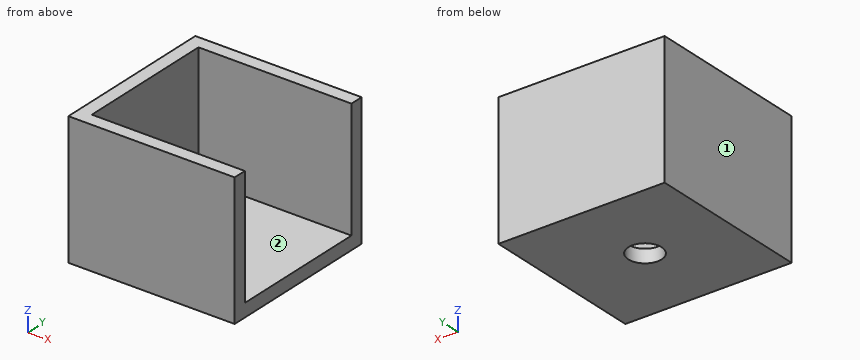
```python
from build123d import *

# Parameters (mm, degrees)
IZIM1_W                     = 25
IZIM1_H                     = 25
Y_KSEKLIK_EKSTR_ZYON1_DEPTH = 20
BO_ALTMA1_T                 = -2
IZIM2_R                     = 2.5
KES_EKSTR_ZYON1_DEPTH       = 5


with BuildPart() as part:
    # Çizim1 → Yükseklik-Ekstrüzyon1 (new body)
    with BuildSketch(Plane.XY):
        Rectangle(IZIM1_W, IZIM1_H)
    extrude(amount=Y_KSEKLIK_EKSTR_ZYON1_DEPTH)

    # İç Boşaltma1
    bo_altma1_openings = [part.faces().sort_by_distance(p)[0] for p in [
        (0, 0, 20),
        (12.5, 0, 10),
    ]]
    offset(amount=BO_ALTMA1_T, openings=bo_altma1_openings, kind=Kind.INTERSECTION)

    # Çizim2 → Kes-Ekstrüzyon1 (cut)
    with BuildSketch(Plane.XY.offset(2)):
        Circle(IZIM2_R)
    extrude(amount=-KES_EKSTR_ZYON1_DEPTH, mode=Mode.SUBTRACT)


solid = part.part
```
Part model, mm, in its own coordinate system. Face numbers are marked on the shaded views. A direction names the side the tool comes from. Give positions to 0.01 mm unless a question says otherwise; leave off trailing zeros. Write each loop counter-clockwise with the first axis right and the second up, starting at its lowest first coordinate (ties: lowest second). Pieces come first, ordered by that corner, then holes. Notation, with made-up numbers: M 39.25,85 L 51.25,85 A13 cw 51.25,105 Z; hole C 75,-25 d7. An arc over 180 degrees is marked long. Use CSV: the item, a comma, the result in double quotes.
Item 1: Slice it at C-C on z = 2.75. Write the cut outline in (x, y).
Taken from the geometry:
outline,"M -12.5,-12.5 L 12.5,-12.5 L 12.5,-10.5 L -10.5,-10.5 L -10.5,10.5 L 12.5,10.5 L 12.5,12.5 L -12.5,12.5 Z"
Item 2: Drill centre lines: probe 1 along Y at (x, z) = (-2, 11.5); probe 2 along Y at (x, z) = (0, 0.55); probe 3 along Z at (x, y) = (6.5, 9.5). Where is each one in solid material? Low to high.
Taken from the geometry:
probe 1,"y = -12.5 to -10.5, 10.5 to 12.5"
probe 2,"y = -12.5 to -2.5, 2.5 to 12.5"
probe 3,"z = 0 to 2"
Item 3: Which spindle directions (+Z, -Z, +X, -X, +Y, -Y) get a long thin tool onto all of the face, cutting with end or side? Do the marked faces 1 and 2. Say none if no direction does.
Taken from the geometry:
face 1,"+Z, -Z, -X, +Y, -Y"
face 2,"+Z, +X"
Item 4: Slice it at B-B on x = 0. Write the cut outline in (y, z), plus the area to 3 significant figures.
Taken from the geometry:
outline,"M -12.5,0 L -2.5,0 L -2.5,2 L -10.5,2 L -10.5,20 L -12.5,20 Z; M 2.5,0 L 12.5,0 L 12.5,20 L 10.5,20 L 10.5,2 L 2.5,2 Z"
area,"112 mm²"
Item 5: Slice it at D-D on y = 8.75. Write the cut outline in (x, z), plus the area to 3 significant figures.
Taken from the geometry:
outline,"M -12.5,0 L 12.5,0 L 12.5,2 L -10.5,2 L -10.5,20 L -12.5,20 Z"
area,"86.0 mm²"
Item 6: Pin check, flat tip, straight feed: P1, Ø9, axis at y = 0.5, z = 14, coming from the +X side. Stop position of the tip, or through.
Taken from the geometry:
P1,"stops at x = -10.5"
Item 7: Slice it at A-A on y = 0. Write the cut outline in (x, z).
Taken from the geometry:
outline,"M -12.5,0 L -2.5,0 L -2.5,2 L -10.5,2 L -10.5,20 L -12.5,20 Z; M 2.5,0 L 12.5,0 L 12.5,2 L 2.5,2 Z"
